from build123d import *

# Parameters (mm, degrees)
SKETCH1_R           = 14.2875
BOSS_EXTRUDE1_DEPTH = 5.842


with BuildPart() as part:
    # Sketch1 → Boss-Extrude1 (new body)
    with BuildSketch(Plane(origin=(0, 0, 0), x_dir=(-1, 0, 0), z_dir=(0, 0, -1))):
        with BuildLine():
            Line((73.788575358, 2.063404121), (73.788575358, 97.70823332))
            Line((73.788575358, 97.70823332), (118.435989957, 175.039823832))
            ThreePointArc((118.435989957, 175.039823832), (110.301075358, 205.399738431), (79.941160759, 197.264823832))
            Line((79.941160759, 197.264823832), (32.316160759, 114.775904121))
            ThreePointArc((32.316160759, 114.775904121), (30.095873869, 109.415657399), (29.338575358, 103.663404121))
            Line((29.338575358, 103.663404121), (29.338575358, 2.063404121))
            ThreePointArc((29.338575358, 2.063404121), (51.563575358, -20.161595879), (73.788575358, 2.063404121))
        make_face()
        with Locations((51.563575358, 2.063404121)):
            Circle(SKETCH1_R, mode=Mode.SUBTRACT)
        with Locations((51.563575358, 103.663404121)):
            Circle(SKETCH1_R, mode=Mode.SUBTRACT)
        with Locations((99.188575358, 186.152323832)):
            Circle(SKETCH1_R, mode=Mode.SUBTRACT)
    extrude(amount=-BOSS_EXTRUDE1_DEPTH)


solid = part.part
Check sheet for the modelled part. Datum: model origin and axes. Units: mm. A direction names the side the tool comes from. Round coordinates to 2 decimals unless told otherwise and drop trailing zeros. Write each loop counter-clockwise with the first axis right and the second up, starting at its lowest first coordinate (ties: lowest second). Pieces come first, ordered by that corner, then holes. Notation, with made-up numbers: (89, 52.5) -> (146, 52.5) arc R18 ccw to (146, 68.5) -> close; hole circle Ø3 at (-28.75, 88.25). An arc over 180 degrees is marked (long way). Answer as CSV lines item,"result". Start each with the question number.
1) Section check B-B on z = 1.45. State how many separate pieces and enclosed holes the cut face has, and give its area (3 significant figures).
2) Release check for a two-part mould opening along X. For faces 1 (the flat face through (-65, 96, 0)), 2 (the cylindrical face through (-64.76, -3.41, 2.88)), 3 (the cylindrical face through (-51.075, -20.156, 2.88)), 4 (the cylindrical face through (-59.244, 115.711, 2.88)) record: pulls with the +X half, pulls with the -X half, needs draft (parallel to the pull), parting line crosses it, or undercut.
3) Material ranges on line 1 (Y direction, x = -48.5, z = 1.4); line 2 (Y direction, x = -60, z = 4.1); line 3 (X direction, y = -2.5, z = 1.45), recorded low to high. Write a range as from..to.
4) Section check C-C on x = -54.5. Enter the section's corners in (y, z).
5) Section check D-D on y = 52. Enter the section's corners in (x, z).
6) Tool access check on faces 5 (the flat face through (-73.789, 49, 3)), 6 (the flat face through (-29.339, 54, 3)). Record the directions out of +Z, -Z, +X, -X, +Y, -Y that give a thin tool (end or side, any length) a straight path to the whole face; none if there is none.
7) Section check A-A on x = -90. Enter the section's corners in (y, z).
Found:
1,separate pieces,"1"
1,enclosed holes,"3"
1,area,"8,370 mm^2"
2,face 1,"needs draft"
2,face 2,"undercut"
2,face 3,"parting line crosses it"
2,face 4,"undercut"
3,line 1,"y = -19.95..-11.89, 16.02..89.71, 117.62..142.81"
3,line 2,"y = -18.5..-9.47, 13.59..92.13, 115.19..162.73"
3,line 3,"x = -73.32..-65.1, -38.02..-29.81"
4,outline,"(-19.97, 0) -> (-11.92, 0) -> (-11.92, 5.84) -> (-19.97, 5.84) -> close; (16.05, 0) -> (89.68, 0) -> (89.68, 5.84) -> (16.05, 5.84) -> close; (117.65, 0) -> (153.2, 0) -> (153.2, 5.84) -> (117.65, 5.84) -> close"
5,outline,"(-73.79, 0) -> (-29.34, 0) -> (-29.34, 5.84) -> (-73.79, 5.84) -> close"
6,face 5,"+Z, -Z, -X, -Y"
6,face 6,"+Z, -Z, +X, +Y, -Y"
7,outline,"(125.79, 0) -> (175.21, 0) -> (175.21, 5.84) -> (125.79, 5.84) -> close; (197.09, 0) -> (206.39, 0) -> (206.39, 5.84) -> (197.09, 5.84) -> close"
